Check sheet for the modelled part. Datum: model origin and axes. Units: mm. Round coordinates to 2 decimals unless told otherwise and drop trailing zeros. Answer in a Markdown table with one row per item.
from build123d import *

# Parameters (mm, degrees)
BOSS_EXTRUDE1_DEPTH = 838.2


with BuildPart() as part:
    # Sketch1 → Boss-Extrude1 (new body)
    with BuildSketch(Plane.XY.offset(838.2)):
        with BuildLine():
            Line((-19.05, 15.875), (-19.05, 9.525))
            ThreePointArc((-19.05, 9.525), (-10.680576272, -10.680576272), (9.525, -19.05))
            Line((9.525, -19.05), (15.875, -19.05))
            ThreePointArc((15.875, -19.05), (18.12006403, -18.12006403), (19.05, -15.875))
            Line((19.05, -15.875), (19.05, -5.6388))
            ThreePointArc((19.05, -5.6388), (18.588751759, -4.525248241), (17.4752, -4.064))
            Line((17.4752, -4.064), (16.5608, -4.064))
            ThreePointArc((16.5608, -4.064), (15.447248241, -4.525248241), (14.986, -5.6388))
            Line((14.986, -5.6388), (14.986, -6.476993142))
            ThreePointArc((14.986, -6.476993142), (15.097592316, -6.746400826), (15.367, -6.857993142))
            Line((15.367, -6.857993142), (15.44319365, -6.857993142))
            ThreePointArc((15.44319365, -6.857993142), (15.712601334, -6.969585458), (15.82419365, -7.238993142))
            Line((15.82419365, -7.238993142), (15.82419365, -9.017))
            ThreePointArc((15.82419365, -9.017), (15.452219262, -9.915025612), (14.55419365, -10.287))
            Line((14.55419365, -10.287), (12.968312693, -10.287))
            ThreePointArc((12.968312693, -10.287), (12.482304734, -10.190327006), (12.070287081, -9.915025612))
            Line((12.070287081, -9.915025612), (8.122184211, -5.966922742))
            ThreePointArc((8.122184211, -5.966922742), (7.092556996, -4.425976719), (6.731, -2.608306952))
            Line((6.731, -2.608306952), (6.731, 2.608306952))
            ThreePointArc((6.731, 2.608306952), (7.092556996, 4.425976719), (8.122184211, 5.966922742))
            Line((8.122184211, 5.966922742), (12.070287081, 9.915025612))
            ThreePointArc((12.070287081, 9.915025612), (12.482304734, 10.190327006), (12.968312693, 10.287))
            Line((12.968312693, 10.287), (14.55419365, 10.287))
            ThreePointArc((14.55419365, 10.287), (15.452219262, 9.915025612), (15.82419365, 9.017))
            Line((15.82419365, 9.017), (15.82419365, 7.238993142))
            ThreePointArc((15.82419365, 7.238993142), (15.712601334, 6.969585458), (15.44319365, 6.857993142))
            Line((15.44319365, 6.857993142), (15.367, 6.857993142))
            ThreePointArc((15.367, 6.857993142), (15.097592316, 6.746400826), (14.986, 6.476993142))
            Line((14.986, 6.476993142), (14.986, 5.6388))
            ThreePointArc((14.986, 5.6388), (15.447248241, 4.525248241), (16.5608, 4.064))
            Line((16.5608, 4.064), (17.4752, 4.064))
            ThreePointArc((17.4752, 4.064), (18.588751759, 4.525248241), (19.05, 5.6388))
            Line((19.05, 5.6388), (19.05, 15.875))
            ThreePointArc((19.05, 15.875), (18.12006403, 18.12006403), (15.875, 19.05))
            Line((15.875, 19.05), (5.6388, 19.05))
            ThreePointArc((5.6388, 19.05), (4.525248241, 18.588751759), (4.064, 17.4752))
            Line((4.064, 17.4752), (4.064, 16.5608))
            ThreePointArc((4.064, 16.5608), (4.525248241, 15.447248241), (5.6388, 14.986))
            Line((5.6388, 14.986), (6.476993142, 14.986))
            ThreePointArc((6.476993142, 14.986), (6.746400826, 15.097592316), (6.857993142, 15.367))
            Line((6.857993142, 15.367), (6.857993142, 15.44319365))
            ThreePointArc((6.857993142, 15.44319365), (6.969585458, 15.712601334), (7.238993142, 15.82419365))
            Line((7.238993142, 15.82419365), (9.017, 15.82419365))
            ThreePointArc((9.017, 15.82419365), (9.915025612, 15.452219262), (10.287, 14.55419365))
            Line((10.287, 14.55419365), (10.287, 12.968312693))
            ThreePointArc((10.287, 12.968312693), (10.190327006, 12.482304734), (9.915025612, 12.070287081))
            Line((9.915025612, 12.070287081), (5.966922742, 8.122184211))
            ThreePointArc((5.966922742, 8.122184211), (4.425976719, 7.092556996), (2.608306952, 6.731))
            Line((2.608306952, 6.731), (-2.608306952, 6.731))
            ThreePointArc((-2.608306952, 6.731), (-4.425976719, 7.092556996), (-5.966922742, 8.122184211))
            Line((-5.966922742, 8.122184211), (-9.915025612, 12.070287081))
            ThreePointArc((-9.915025612, 12.070287081), (-10.190327006, 12.482304734), (-10.287, 12.968312693))
            Line((-10.287, 12.968312693), (-10.287, 14.55419365))
            ThreePointArc((-10.287, 14.55419365), (-9.915025612, 15.452219262), (-9.017, 15.82419365))
            Line((-9.017, 15.82419365), (-7.238993142, 15.82419365))
            ThreePointArc((-7.238993142, 15.82419365), (-6.969585458, 15.712601334), (-6.857993142, 15.44319365))
            Line((-6.857993142, 15.44319365), (-6.857993142, 15.367))
            ThreePointArc((-6.857993142, 15.367), (-6.746400826, 15.097592316), (-6.476993142, 14.986))
            Line((-6.476993142, 14.986), (-5.6388, 14.986))
            ThreePointArc((-5.6388, 14.986), (-4.525248241, 15.447248241), (-4.064, 16.5608))
            Line((-4.064, 16.5608), (-4.064, 17.4752))
            ThreePointArc((-4.064, 17.4752), (-4.525248241, 18.588751759), (-5.6388, 19.05))
            Line((-5.6388, 19.05), (-15.875, 19.05))
            ThreePointArc((-15.875, 19.05), (-18.12006403, 18.12006403), (-19.05, 15.875))
        make_face()
        with BuildLine():
            Line((-14.4526, 17.2466), (-12.2428, 17.2466))
            ThreePointArc((-12.2428, 17.2466), (-11.973392316, 17.135007684), (-11.8618, 16.8656))
            Line((-11.8618, 16.8656), (-11.8618, 12.2428))
            ThreePointArc((-11.8618, 12.2428), (-11.973392316, 11.973392316), (-12.2428, 11.8618))
            Line((-12.2428, 11.8618), (-16.8656, 11.8618))
            ThreePointArc((-16.8656, 11.8618), (-17.135007684, 11.973392316), (-17.2466, 12.2428))
            Line((-17.2466, 12.2428), (-17.2466, 14.4526))
            ThreePointArc((-17.2466, 14.4526), (-16.428256347, 16.428256347), (-14.4526, 17.2466))
        make_face(mode=Mode.SUBTRACT)
        with BuildLine():
            Line((-14.726680045, 10.287), (-12.804003164, 10.287))
            ThreePointArc((-12.804003164, 10.287), (-12.463797593, 10.219328904), (-12.175385236, 10.026617928))
            Line((-12.175385236, 10.026617928), (-6.696574388, 4.547807081))
            ThreePointArc((-6.696574388, 4.547807081), (-6.421272994, 4.135789428), (-6.3246, 3.649781469))
            Line((-6.3246, 3.649781469), (-6.3246, 0))
            ThreePointArc((-6.3246, 0), (-4.472167548, -4.472167548), (0, -6.3246))
            Line((0, -6.3246), (3.649781469, -6.3246))
            ThreePointArc((3.649781469, -6.3246), (4.135789428, -6.421272994), (4.547807081, -6.696574388))
            Line((4.547807081, -6.696574388), (10.026617928, -12.175385236))
            ThreePointArc((10.026617928, -12.175385236), (10.219328904, -12.463797593), (10.287, -12.804003164))
            Line((10.287, -12.804003164), (10.287, -14.726680045))
            ThreePointArc((10.287, -14.726680045), (9.905572448, -15.634060343), (8.990403141, -15.996401513))
            ThreePointArc((8.990403141, -15.996401513), (-8.525314803, -8.525314803), (-15.996401513, 8.990403141))
            ThreePointArc((-15.996401513, 8.990403141), (-15.634060343, 9.905572448), (-14.726680045, 10.287))
        make_face(mode=Mode.SUBTRACT)
        with BuildLine():
            Line((-3.437208141, -1.820762039), (-3.017877069, -1.401430967))
            ThreePointArc((-3.017877069, -1.401430967), (-3.3274, 0), (-3.017877069, 1.401430967))
            Line((-3.017877069, 1.401430967), (-3.437208141, 1.820762039))
            ThreePointArc((-3.437208141, 1.820762039), (-3.437208141, 3.437208141), (-1.820762039, 3.437208141))
            Line((-1.820762039, 3.437208141), (-1.401430967, 3.017877069))
            ThreePointArc((-1.401430967, 3.017877069), (0, 3.3274), (1.401430967, 3.017877069))
            Line((1.401430967, 3.017877069), (1.820762039, 3.437208141))
            ThreePointArc((1.820762039, 3.437208141), (3.437208141, 3.437208141), (3.437208141, 1.820762039))
            Line((3.437208141, 1.820762039), (3.017877069, 1.401430967))
            ThreePointArc((3.017877069, 1.401430967), (3.3274, 0), (3.017877069, -1.401430967))
            Line((3.017877069, -1.401430967), (3.437208141, -1.820762039))
            ThreePointArc((3.437208141, -1.820762039), (3.437208141, -3.437208141), (1.820762039, -3.437208141))
            Line((1.820762039, -3.437208141), (1.401430967, -3.017877069))
            ThreePointArc((1.401430967, -3.017877069), (0, -3.3274), (-1.401430967, -3.017877069))
            Line((-1.401430967, -3.017877069), (-1.820762039, -3.437208141))
            ThreePointArc((-1.820762039, -3.437208141), (-3.437208141, -3.437208141), (-3.437208141, -1.820762039))
        make_face(mode=Mode.SUBTRACT)
        with BuildLine():
            Line((12.2428, 17.2466), (14.4526, 17.2466))
            ThreePointArc((14.4526, 17.2466), (16.428256347, 16.428256347), (17.2466, 14.4526))
            Line((17.2466, 14.4526), (17.2466, 12.2428))
            ThreePointArc((17.2466, 12.2428), (17.135007684, 11.973392316), (16.8656, 11.8618))
            Line((16.8656, 11.8618), (12.2428, 11.8618))
            ThreePointArc((12.2428, 11.8618), (11.973392316, 11.973392316), (11.8618, 12.2428))
            Line((11.8618, 12.2428), (11.8618, 16.8656))
            ThreePointArc((11.8618, 16.8656), (11.973392316, 17.135007684), (12.2428, 17.2466))
        make_face(mode=Mode.SUBTRACT)
        with BuildLine():
            Line((11.8618, -16.8656), (11.8618, -12.2428))
            ThreePointArc((11.8618, -12.2428), (11.973392316, -11.973392316), (12.2428, -11.8618))
            Line((12.2428, -11.8618), (16.8656, -11.8618))
            ThreePointArc((16.8656, -11.8618), (17.135007684, -11.973392316), (17.2466, -12.2428))
            Line((17.2466, -12.2428), (17.2466, -14.4526))
            ThreePointArc((17.2466, -14.4526), (16.428256347, -16.428256347), (14.4526, -17.2466))
            Line((14.4526, -17.2466), (12.2428, -17.2466))
            ThreePointArc((12.2428, -17.2466), (11.973392316, -17.135007684), (11.8618, -16.8656))
        make_face(mode=Mode.SUBTRACT)
    extrude(amount=-BOSS_EXTRUDE1_DEPTH)


solid = part.part
Item 1: Depth check by flat-ended pin: P1, Ø1, axis at x = 17, z = 413, coming from the +Y side; P2, Ø4, axis at y = -1, z = 388.5, coming from the +X side; P3, Ø2.5, axis at x = -0.5, z = 514.5, coming from the +Y side. Enter the tip coordinate at first touch or a pass-through.
Result sheet:
| item | result |
|---|---|
| P1 | stops at y = 18.99 |
| P2 | stops at x = 6.75 |
| P3 | stops at y = 6.73 |
Item 2: Scan lines: line 1 (X direction, y = 14, z = 565.5); line 2 (Y direction, x = -5.5, z = 780); line 3 (X direction, y = -14, z = 216.5). Record each from-to range of solid material in increasing order. Write a range as [from, to].
Result sheet:
| item | result |
|---|---|
| line 1 | x = [-19.05, -17.25], [-11.86, -10.29], [10.29, 11.86], [17.25, 19.05] |
| line 2 | y = [-14.78, -11.11], [-3.12, 7.71], [14.99, 19.04] |
| line 3 | x = [-6.7, -0.38], [10.29, 11.86], [17.25, 19.05] |
Item 3: Mould release check, pull along X, two halves, no side actions. Record for faces 1 (the cylindrical face through (-8.33, -8.72, 424.97)), 2 (the flat face through (4, 2, 838.2)), 3 (the cylindrical face through (-10.9, -10.46, 424.97)): pulls with the +X half, pulls with the -X half, needs draft (parallel to the pull), parting line crosses it, or undercut.
Result sheet:
| item | result |
|---|---|
| face 1 | undercut |
| face 2 | needs draft |
| face 3 | pulls with the -X half |
Item 4: Cross-section at A-A (z = 605.5). State how many separate pieces and enclosed holes the cut face has, and give its area (3 significant figures).
Result sheet:
| item | result |
|---|---|
| separate pieces | 1 |
| enclosed holes | 5 |
| area | 542 mm^2 |
